from build123d import *

# Parameters (mm, degrees)
SKETCH1_W             = 60
SKETCH1_H             = 50
BOSS_EXTRUDE1_DEPTH   = 10
M3_TAPPED_HOLE1_D     = 2.5
M3_TAPPED_HOLE1_DEPTH = 10
CUT_EXTRUDE1_DEPTH    = 6.4
CUT_EXTRUDE2_DEPTH    = 4.6
FILLET1_R             = 2.5


with BuildPart() as part:
    # Sketch1 → Boss-Extrude1 (new body)
    with BuildSketch(Plane(origin=(0, 0, 0), x_dir=(1, 0, 0), z_dir=(0, 1, 0))):
        Rectangle(SKETCH1_W, SKETCH1_H)
    extrude(amount=BOSS_EXTRUDE1_DEPTH)

    # M3 Tapped Hole1
    with Locations(Plane(origin=(0, 10, 0), x_dir=(1, 0, 0), z_dir=(0, 1, 0))):
        with Locations((-23.4, 6.6), (23.4, 2.8)):
            Hole(M3_TAPPED_HOLE1_D / 2, depth=M3_TAPPED_HOLE1_DEPTH)

    # Sketch7 → Cut-Extrude1 (cut)
    with BuildSketch(Plane(origin=(0, 10, 0), x_dir=(1, 0, 0), z_dir=(0, 1, 0))):
        with BuildLine():
            Line((-22.5, 23), (22.5, 23))
            ThreePointArc((22.5, 23), (28, 17.5), (22.5, 12))
            Line((22.5, 12), (-22.5, 12))
            ThreePointArc((-22.5, 12), (-28, 17.5), (-22.5, 23))
        make_face()
    extrude(amount=-CUT_EXTRUDE1_DEPTH, mode=Mode.SUBTRACT)

    # Sketch8 → Cut-Extrude2 (cut, through all)
    with BuildSketch(Plane(origin=(0, 3.6, 0), x_dir=(1, 0, 0), z_dir=(0, 1, 0))):
        with BuildLine():
            Line((-22.5, 20.7), (22.5, 20.7))
            ThreePointArc((22.5, 20.7), (25.7, 17.5), (22.5, 14.3))
            Line((22.5, 14.3), (-22.5, 14.3))
            ThreePointArc((-22.5, 14.3), (-25.7, 17.5), (-22.5, 20.7))
        make_face()
    extrude(amount=-CUT_EXTRUDE2_DEPTH, mode=Mode.SUBTRACT)

    # Fillet1
    fillet1_edges = [part.edges().sort_by_distance(p)[0] for p in [
        (30, 5, 25),
        (-30, 5, 25),
        (-30, 5, -25),
        (30, 5, -25),
    ]]
    fillet(fillet1_edges, radius=FILLET1_R)


solid = part.part
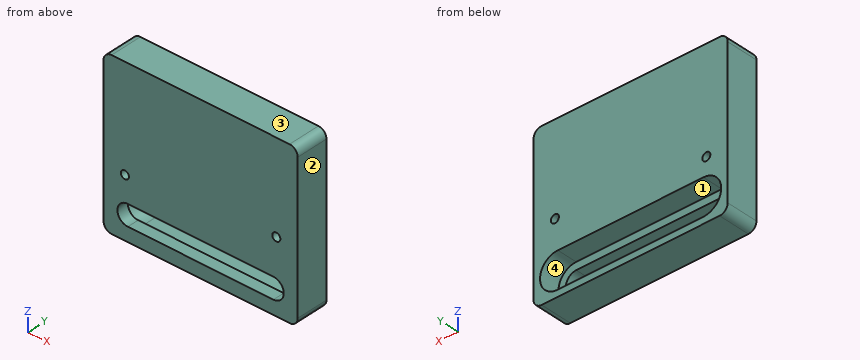
Can you work these out from the model? Positions are in its coordinate system, mm. Face numbers are marked on the shaded views. Give positions to 0.01 mm unless a question says otherwise; leave off trailing zeros. Loops run counter-clockwise (first coordinate to the right, second up) from the corner with the lowest first, then second, coordinate; pieces in that order, holes last. Notation, with made-up numbers: (56, -2.75) -> (69, -2.75) arc R21 ccw to (69, 6.25) -> close; hole circle Ø5 at (-29.5, 24). An arc over 180 degrees is marked (long way). Use one line per item in the form item = value.
1) We'd pull the mould along Z, two halves only. Please class the marked faces 1, 2, 3 and 4: released by +Z, released by -Z, zero draft, split by the parting line, or undercut.
Answers:
face_1 = undercut
face_2 = zero draft
face_3 = released by +Z
face_4 = undercut
2) If we section it at B-B (z = -2.8): Please give me the cut outline in (x, y).
Answers:
outline = (-30, 0) -> (22.15, 0) -> (22.15, 10) -> (-30, 10) -> close; (24.65, 0) -> (30, 0) -> (30, 10) -> (24.65, 10) -> close
3) If we section it at D-D (x = -23.4): Please give me the cut outline in (y, z), plus the area to 3 significant figures.
Answers:
outline = (0, -25) -> (10, -25) -> (10, -22.93) -> (3.6, -22.93) -> (3.6, -20.57) -> (0, -20.57) -> close; (0, -14.43) -> (3.6, -14.43) -> (3.6, -12.07) -> (10, -12.07) -> (10, -7.85) -> (0, -7.85) -> close; (0, -5.35) -> (10, -5.35) -> (10, 25) -> (0, 25) -> close
area = 383 mm²
4) I need wall thicknesses on line 1 along Z through (x, y) = (3.5, 1.5); line 2 along Z through (x, y) = (-23.4, 5.75); line 3 along Z through (x, y) = (21.5, 8). Which ranges of each line are inside material? Lowest first, please.
Answers:
line_1 = -25 to -20.7, -14.3 to 25
line_2 = -25 to -22.93, -12.07 to -7.85, -5.35 to 25
line_3 = -25 to -23, -12 to 25
5) If we section it at C-C (y = 6.75): Please give me the cut outline in (x, z), plus the area to 3 significant figures.
Answers:
outline = (-30, -22.5) arc R2.5 ccw to (-27.5, -25) -> (27.5, -25) arc R2.5 ccw to (30, -22.5) -> (30, 22.5) arc R2.5 ccw to (27.5, 25) -> (-27.5, 25) arc R2.5 ccw to (-30, 22.5) -> close; hole circle Ø2.5 at (-23.4, -6.6); hole (-22.5, -23) -> (22.5, -23) arc R5.5 ccw to (22.5, -12) -> (-22.5, -12) arc R5.5 ccw to start; hole circle Ø2.5 at (23.4, -2.8)
area = 2,390 mm²
6) If we section it at A-A (x = -16): Please give me the cut outline in (y, z), plus the area to 3 significant figures.
Answers:
outline = (0, -25) -> (10, -25) -> (10, -23) -> (3.6, -23) -> (3.6, -20.7) -> (0, -20.7) -> close; (0, -14.3) -> (3.6, -14.3) -> (3.6, -12) -> (10, -12) -> (10, 25) -> (0, 25) -> close
area = 407 mm²
